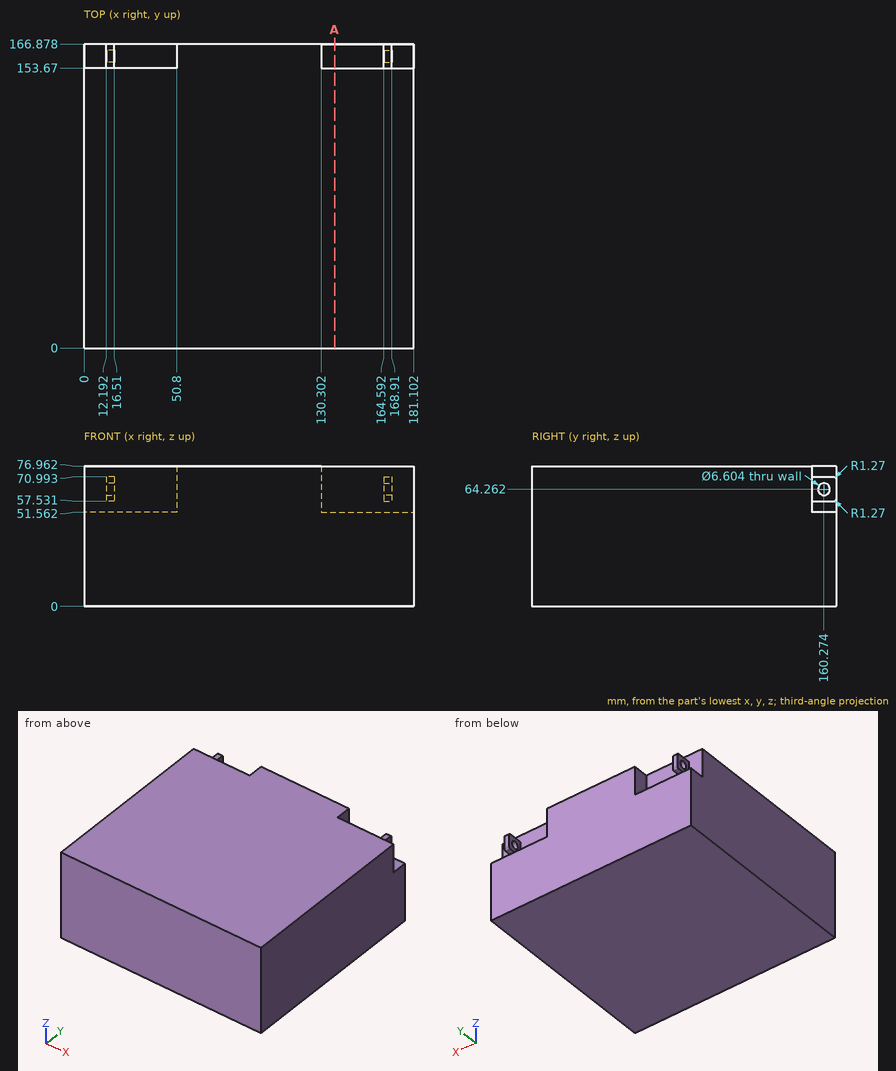
Geometry check sheet. Reference: drawing and pictorial views, mm from the part's lowest x, y, z. Coordinates: 2 decimals unless noted, no trailing zeros. Write each loop counter-clockwise with the first axis right and the second up, starting at its lowest first coordinate (ties: lowest second). Pieces come first, ordered by that corner, then holes. Notation, with made-up numbers: (57, -4) - (111, -4) arc R19 ccw to (111, 10) - close; hole circle Ø6 at (30, 71). An arc over 180 degrees is marked (long way). One line per question, with ' | ' between items. Start each with the question number.
1. Gauge pin test, flat ends, axial feed: P1, Ø4, axis at y = 160, z = 66, coming from the +X side; P2, Ø4, axis at y = 163.5, z = 61, coming from the -X side; P3, Ø4, axis at y = 160.274, z = 64.262, coming from the -X side. Record the tip position at first contact, or that the pin passes through.
2. Section check A-A (x = 137.5). Enter the section's corners in (y, z).
3. Material ranges on line 1 along Y through (x, z) = (11, 54), recorded low to high.
Computed values:
1) P1: x = 168.91 | P2: x = 12.19 | P3: x = 50.8
2) outline: (0, 0) - (166.88, 0) - (166.88, 51.56) - (153.67, 51.56) - (153.67, 76.96) - (0, 76.96) - close
3) line 1: 0 to 153.67
